```python
from build123d import *

# Parameters (mm, degrees)
F0_W     = 6.35
F0_H     = 127
F1_DEPTH = 25.4
F2_R     = 12.69999
F3_W     = 6.35
F3_H     = 25.3775035135
F4_DEPTH = 38.1
F5_R     = 3.17499
F6_R     = 4.7625
F7_DEPTH = 25.4


# Not quite as in the source:
# - a fillet or chamfer is up to 0.001 mm smaller than in the source, because OpenCascade refuses the exact size


with BuildPart() as f1:
    # F0 (on Front) → F1 (new body)
    with BuildSketch(Plane.XZ):
        with Locations((3.175, 63.5)):
            Rectangle(F0_W, F0_H)
    extrude(amount=F1_DEPTH)

    # F2 (radius 12.7 in the source; OpenCascade refuses exactly that, so slightly less here)
    f2_edges = [f1.edges().sort_by_distance(p)[0] for p in [
        (3.175, -25.4, 127),
        (3.175, 0, 127),
    ]]
    fillet(f2_edges, radius=F2_R)

    # F3 (on face) → F4 (join)
    with BuildSketch(Plane.YZ.offset(6.35)):
        with Locations((-12.7, 107.9612482432)):
            Rectangle(F3_W, F3_H)
    extrude(amount=F4_DEPTH)

    # F5 (radius 3.175 in the source; OpenCascade refuses exactly that, so slightly less here)
    f5_edges = [f1.edges().sort_by_distance(p)[0] for p in [
        (25.4, -15.875, 120.65),
        (25.4, -9.525, 120.65),
        (25.4, -15.875, 95.272496),
        (25.4, -9.525, 95.272496),
        (44.45, -15.875, 107.961248),
        (44.45, -9.525, 107.961248),
        (44.45, -12.7, 95.272496),
        (44.45, -12.7, 120.65),
    ]]
    fillet(f5_edges, radius=F5_R)

    # F6 (on face) → F7 (cut)
    with BuildSketch(Plane.XZ.offset(15.875)):
        with Locations((23.8125, 107.9612482432)):
            Circle(F6_R)
    extrude(amount=-F7_DEPTH, mode=Mode.SUBTRACT)


solid = f1.part
```
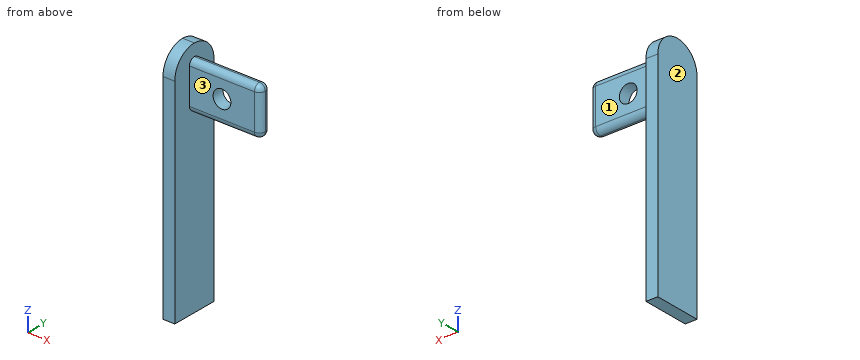
The listing builds one solid part. Answer for the finished solid, in the listing's coordinates (mm). Face numbers are marked on the shaded views. A direction names the side the tool comes from. Give positions to 0.01 mm unless a question says otherwise; leave off trailing zeros.
1) For the marked faces 1, 2 and 3, determine the directions among +Z, -Z, +X, -X, +Y, -Y from which every point of the face is accessible in a straight line to the end or side of a thin tool.
Reported:
face 1: +Z, -Z, +X, +Y
face 2: +Z, -Z, -X, +Y, -Y
face 3: +Z, -Z, +X, -Y
2) Given P1, Ø5.5, axis at x = 32, z = 107, coming from the +Y side (3 decimals); P2, Ø15, axis at x = 23.5, z = 112.5, coming from the -Y side (3 decimals); P3, Ø4, axis at x = 9, z = 70, coming from the -Y side; P4, Ø1.5, axis at y = -4.5, z = 70, coming from the +X side, each flat-ended and moving along its own axis, determine where each tip first touches the part or whether it passes through.
Reported:
P1: stops at y = -9.525
P2: stops at y = -15.875
P3: passes through
P4: stops at x = 6.35
3) Consider line 1 along X through (y, z) = (-16.25, 45); line 2 along Y through (x, z) = (27, 112.5) (3 decimals); line 3 along Z through (x, y) = (14, -13). Determine where each line is inside the solid, lowest interval first.
Reported:
line 1: x = 0 to 6.35
line 2: y = -15.875 to -9.525
line 3: z = 95.29 to 120.64
